Could you check a few things on this drawing? It's one solid part, dimensions in mm from its lowest x, y, z. Round coordinates to 2 decimals unless told otherwise and drop trailing zeros. Write each loop counter-clockwise with the first axis right and the second up, starting at its lowest first coordinate (ties: lowest second). Pieces come first, ordered by that corner, then holes. Notation, with made-up numbers: (20.25, -8.5) -> (60.25, -8.5) arc R29 ccw to (60.25, 21.5) -> close; hole circle Ø1 at (76.25, 78.25). An arc over 180 degrees is marked (long way). Answer as CSV lines item,"result".
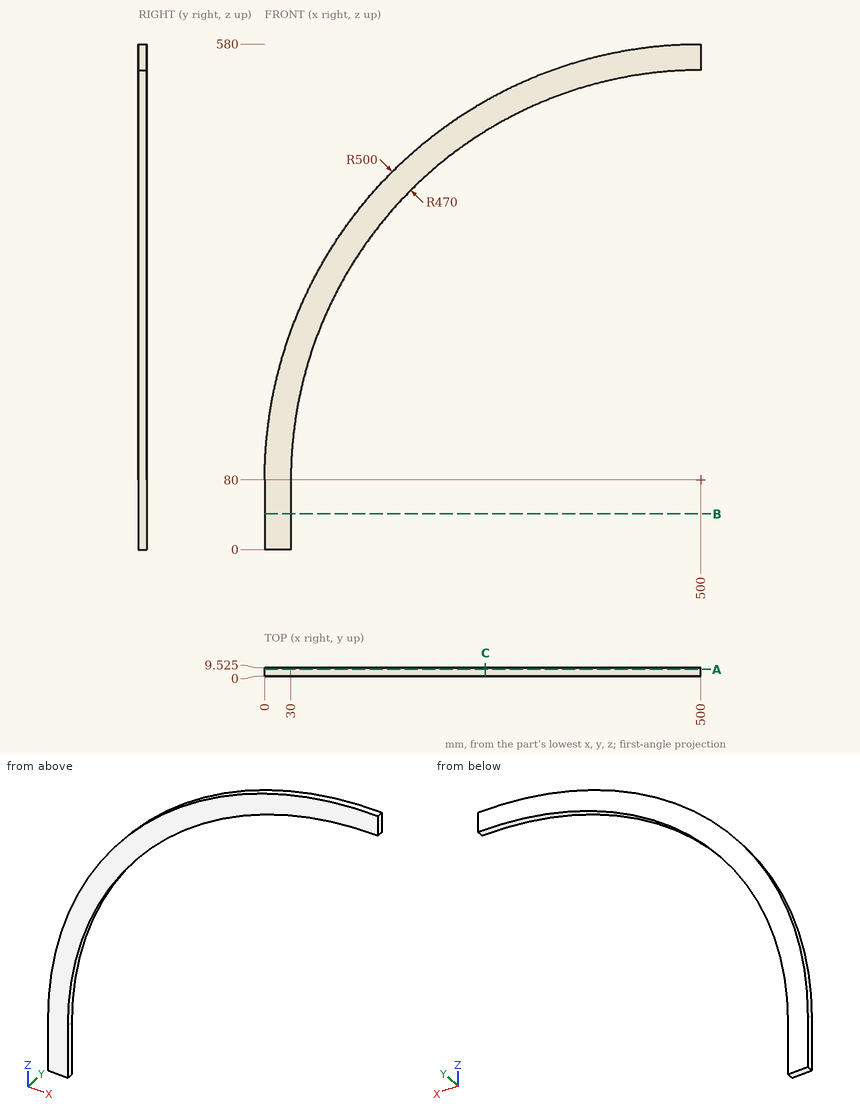
1. Suppose I cut it at A-A on y = 7.5. Please give me the cut outline in (x, z), and give its area (3 significant figures).
Numbers:
outline,"(0, 0) -> (30, 0) -> (30, 80) arc R470 cw to (500, 550) -> (500, 580) arc R500 ccw to (0, 80) -> close"
area,"25,300 mm^2"
2. For pin 1 Ø5 at (y, z) = (7, 56.5) entering from +X; pin 2 Ø4 at (y, z) = (2.5, 418.5) entering from -X; pin 3 Ø4 at (y, z) = (7.5, 491) entering from -X, each with a flat end and sliding along its axis, tell me the tip position at first contact or that it passes through.
Numbers:
pin 1,"stops at x = 30"
pin 2,"stops at x = 130.18"
pin 3,"stops at x = 212.39"
3. Suppose I cut it at B-B on z = 41. Please give me the cut outline in (x, y) (3 decimals), and give its area (3 significant figures).
Numbers:
outline,"(0, 0) -> (30, 0) -> (30, 9.525) -> (0, 9.525) -> close"
area,"286 mm^2"
4. If I drill on line 1 (X direction, y = 2.5, z = 35.5); line 2 (X direction, y = 6.75, z = 363.5); line 3 (Z direction, x = 427.5, y = 6.5), over which ranges is the centre line in solid material (lowest first)?
Numbers:
line 1,"x = 0 to 30"
line 2,"x = 88.14 to 125.13"
line 3,"z = 544.37 to 574.72"
5. Suppose I cut it at C-C on x = 253. Please give me the cut outline in (y, z) (3 decimals).
Numbers:
outline,"(0, 479.864) -> (9.525, 479.864) -> (9.525, 514.731) -> (0, 514.731) -> close"
